Verification items for the finished model (mm, model axes). A direction names the side the tool comes from. Give positions to 0.01 mm unless a question says otherwise; leave off trailing zeros. Write each loop counter-clockwise with the first axis right and the second up, starting at its lowest first coordinate (ties: lowest second). Pieces come first, ordered by that corner, then holes. Notation, with made-up numbers: (-4.5, 11) -> (15.5, 11) arc R29 ccw to (15.5, 31) -> close; hole circle Ø6 at (46, 17). An arc over 180 degrees is marked (long way). Use CSV: the item, a comma, the result in double quotes. Start each with the question number.
```python
from build123d import *

# Parameters (mm, degrees)
F1_DEPTH = 76.2
F2_R     = 7.62
F3_DEPTH = 50.8


with BuildPart() as f1:
    # F0 (on Right) → F1 (new body)
    with BuildSketch(Plane.YZ):
        Polygon((-101.6, 0), (0, 0), (0, 57.15), (-12.7, 57.15), (-12.7, 44.481661), (-12.7, 44.45), (-57.15, 44.45), (-101.6, 36.612266), align=None)
    extrude(amount=-F1_DEPTH)

    # F2 (on Top) → F3 (cut)
    with BuildSketch(Plane.XY):
        with Locations((-20.0025, -67.6275)):
            Circle(F2_R)
    extrude(amount=F3_DEPTH, mode=Mode.SUBTRACT)


solid = f1.part
```
(1) Section check A-A on x = -16.5. Record the cut outline in (y, z).
(2) Section check C-C on z = 26.5. Record the cut outline in (x, y), then the cut area to 3 significant figures.
(3) Thickness scan on line 1 (Y direction, x = -71, z = 47.5); line 2 (X direction, y = -74, z = 6); line 3 (Z direction, x = -39, y = -31). Record the ranges inside material, lowest first. Write a range as from..to.
(4) Section check D-D on y = -55. Record the cut outline in (x, z), then the cut area to 3 significant figures.
(5) Go/stop test with flat-tipped pins: pin 1 (10 mm diameter, centred on x = -66, y = -63.5, fed in from -Z); pin 2 (10 mm diameter, centred on x = -58, y = -77, fed in from +Z); pin 3 (5 mm diameter, centred on x = -57, y = -31, fed in from +Z); pin 4 (6.5 mm diameter, centred on x = -36, z = 49.5, fed in from -Y). Record where each tip stops, or that it passes through.
(6) Draft check along X on faces 1 (the face through (-21.654, -75.066, 21.665)), 2 (the face through (-38, -6, 57.15)), 3 (the face through (-76.2, -52, 23)). Enter one of: released by +X, released by -X, zero draft, split by the parting line, or undercut.
(7) Set-up check for faces 4 (the face through (0, -52, 23)), 5 (the face through (-38, -12.7, 51)): record each of +Z, -Z, +X, -X, +Y, -Y from which the full face is reachable in a straight line by a thin tool's end or side.
(8) Section check B-B on x = -50. Record the cut outline in (y, z), then the cut area to 3 significant figures.
Data:
1,outline,"(-101.6, 0) -> (-74.39, 0) -> (-74.39, 41.41) -> (-101.6, 36.61) -> close; (-60.86, 0) -> (0, 0) -> (0, 57.15) -> (-12.7, 57.15) -> (-12.7, 44.45) -> (-57.15, 44.45) -> (-60.86, 43.8) -> close"
2,outline,"(-76.2, -101.6) -> (0, -101.6) -> (0, 0) -> (-76.2, 0) -> close; hole circle Ø15.24 at (-20, -67.63)"
2,area,"7,560 mm2"
3,line 1,"y = -12.7..0"
3,line 2,"x = -76.2..-24.18, -15.82..0"
3,line 3,"z = 0..44.45"
4,outline,"(-76.2, 0) -> (0, 0) -> (0, 44.45) -> (-76.2, 44.45) -> close"
4,area,"3,390 mm2"
5,pin 1,"stops at z = 0"
5,pin 2,"stops at z = 41.83"
5,pin 3,"stops at z = 44.45"
5,pin 4,"stops at y = -12.7"
6,face 1,"undercut"
6,face 2,"zero draft"
6,face 3,"released by -X"
7,face 4,"+Z, -Z, +X, +Y, -Y"
7,face 5,"+Z, +X, -X, -Y"
8,outline,"(-101.6, 0) -> (0, 0) -> (0, 57.15) -> (-12.7, 57.15) -> (-12.7, 44.45) -> (-57.15, 44.45) -> (-101.6, 36.61) -> close"
8,area,"4,500 mm2"
